The listing builds one solid part. Answer for the finished solid, in the listing's coordinates (mm). Face numbers are marked on the shaded views. A direction names the side the tool comes from. Round coordinates to 2 decimals unless told otherwise and drop trailing zeros. Loops run counter-clockwise (first coordinate to the right, second up) from the corner with the lowest first, then second, coordinate; pieces in that order, holes last. Notation, with made-up numbers: M 65.25,20.5 L 88.25,20.5 A20 cw 88.25,40.5 Z; hole C -7,42 d4. An arc over 180 degrees is marked long. Put each result on its own line as item: value. Start each with the question number.
(1) Flat-ended cylindrical pins translate along their axes: P1, Ø10, axis at x = 25.4, z = -25.4, coming from the -Y side; P2, Ø20, axis at x = 25.4, z = -25.4, coming from the +Y side. Find the tip coordinate at first contact, or state that the pin passes through.
(2) Straight lines are drawn through the part: line 1 (Z direction, x = 25.4, y = 10.5); line 2 (X direction, y = 10, z = -25.4); line 3 (X direction, y = 22, z = -25.4). For each, find the intervals that lie inside material, in ascending order.
(3) Section A-A, the plane z = -25.4 is taken. Determine the outline of the cut face in (x, y), then the cut area to 3 significant figures.
(4) Determine the mould class of the marked faces 3, 4, 5 and 6 for opening direction X: released by +X, released by -X, zero draft, split by the parting line, or undercut.
(5) Section B-B, the plane x = 25.4 is taken. Determine the outline of the cut face in (y, z), then the cut area to 3 significant figures.
(6) Section D-D, the plane z = -16.5 is taken. Determine the outline of the cut face in (x, y), then the cut area to 3 significant figures.
(7) Section C-C, the plane y = 11.75 is taken. Determine the outline of the cut face in (x, z), then the cut area to 3 significant figures.
(8) Which of the six approach directions +Z, -Z, +X, -X, +Y, -Y give full straight-line access (tool end or side, diameter ignored) to the marked faces 1 and 2?
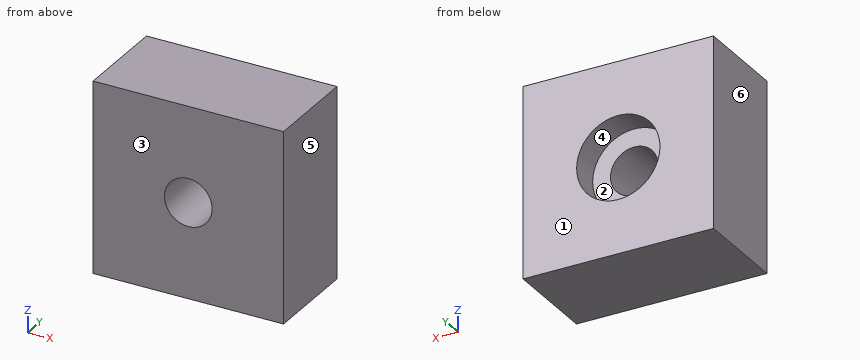
```python
from build123d import *

# Parameters (mm, degrees)
SKETCH1_W           = 50.8
SKETCH1_H           = 50.8
BOSS_EXTRUDE1_DEPTH = 25.4
SKETCH6_R           = 6.35
CUT_EXTRUDE1_DEPTH  = 25.4
SKETCH7_R           = 11.1125
CUT_EXTRUDE2_DEPTH  = 7.62


with BuildPart() as part:
    # Sketch1 → Boss-Extrude1 (new body)
    with BuildSketch(Plane(origin=(0, 0, 0), x_dir=(1, 0, 0), z_dir=(0, 1, 0))):
        with Locations((25.4, 25.4)):
            Rectangle(SKETCH1_W, SKETCH1_H)
    extrude(amount=BOSS_EXTRUDE1_DEPTH)

    # Sketch6 → Cut-Extrude1 (cut)
    with BuildSketch(Plane(origin=(0, 25.4, 0), x_dir=(1, 0, 0), z_dir=(0, 1, 0))):
        with Locations((25.4, 25.4)):
            Circle(SKETCH6_R)
    extrude(amount=-CUT_EXTRUDE1_DEPTH, mode=Mode.SUBTRACT)

    # Sketch7 → Cut-Extrude2 (cut)
    with BuildSketch(Plane(origin=(0, 25.4, 0), x_dir=(1, 0, 0), z_dir=(0, 1, 0))):
        with Locations((25.4, 25.4)):
            Circle(SKETCH7_R)
    extrude(amount=-CUT_EXTRUDE2_DEPTH, mode=Mode.SUBTRACT)


solid = part.part
```
Recorded:
1. P1: passes through
1. P2: stops at y = 17.78
2. line 1: z = -50.8 to -31.75, -19.05 to 0
2. line 2: x = 0 to 19.05, 31.75 to 50.8
2. line 3: x = 0 to 14.29, 36.51 to 50.8
3. outline: M 0,0 L 19.05,0 L 19.05,17.78 L 14.29,17.78 L 14.29,25.4 L 0,25.4 Z; M 31.75,0 L 50.8,0 L 50.8,25.4 L 36.51,25.4 L 36.51,17.78 L 31.75,17.78 Z
3. area: 895 mm²
4. face 3: zero draft
4. face 4: undercut
4. face 5: released by +X
4. face 6: released by -X
5. outline: M 0,-50.8 L 25.4,-50.8 L 25.4,-36.51 L 17.78,-36.51 L 17.78,-31.75 L 0,-31.75 Z; M 0,-19.05 L 17.78,-19.05 L 17.78,-14.29 L 25.4,-14.29 L 25.4,0 L 0,0 Z
5. area: 895 mm²
6. outline: M 0,0 L 50.8,0 L 50.8,25.4 L 32.05,25.4 L 32.05,17.78 L 18.75,17.78 L 18.75,25.4 L 0,25.4 Z
6. area: 1,190 mm²
7. outline: M 0,-50.8 L 50.8,-50.8 L 50.8,0 L 0,0 Z; hole C 25.4,-25.4 d12.7
7. area: 2,450 mm²
8. face 1: +Z, -Z, +X, -X, +Y
8. face 2: +Y
